Verification items for the finished model (mm, model axes). Face numbers are marked on the shaded views. A direction names the side the tool comes from. Coordinates: 2 decimals unless noted, no trailing zeros. Write each loop counter-clockwise with the first axis right and the second up, starting at its lowest first coordinate (ties: lowest second). Pieces come first, ordered by that corner, then holes. Notation, with made-up numbers: (50.25, -23.5) -> (106.25, -23.5) arc R25 ccw to (106.25, 4.5) -> close; hole circle Ø11 at (63, 11). An arc over 180 degrees is marked (long way). Answer in a Markdown table with one row per item.
```python
from build123d import *

# Parameters (mm, degrees)
SKETCH_1_R      = 5
SKETCH_1_R_2    = 3
EXTRUDE_1_DEPTH = 3
EXTRUDE_START   = -0.6
SKETCH_2_R      = 5.6
SKETCH_2_R_2    = 3
EXTRUDE_2_DEPTH = 0.6
FILLET_1_R      = 0.1


with BuildPart() as part:
    # ｽｹｯﾁ1 → ﾎﾞｽ - 押し出し1 (new body)
    with BuildSketch(Plane.XY):
        Circle(SKETCH_1_R)
        Circle(SKETCH_1_R_2, mode=Mode.SUBTRACT)
    extrude(amount=EXTRUDE_1_DEPTH)

    # ｽｹｯﾁ2 → ﾎﾞｽ - 押し出し2 (add)
    with BuildSketch(Plane.XY.offset(3).offset(EXTRUDE_START)):
        Circle(SKETCH_2_R)
        Circle(SKETCH_2_R_2, mode=Mode.SUBTRACT)
    extrude(amount=EXTRUDE_2_DEPTH)

    # ﾌｨﾚｯﾄ1
    fillet_1_edges = [part.edges().sort_by_distance(p)[0] for p in [
        (-5, 0, 0),
        (-3, 0, 0),
        (-3, 0, 3),
    ]]
    fillet(fillet_1_edges, radius=FILLET_1_R)


solid = part.part
```
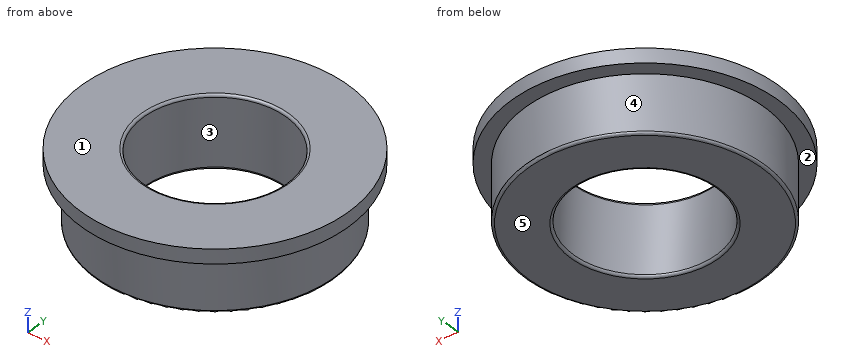
1. Sectioned sample at C-C, the plane z = 2.55. Record the cut outline in (x, y).
Findings below:
| item | result |
|---|---|
| outline | circle Ø11.2 at (0, 0); hole circle Ø6 at (0, 0) |
2. Access from +Z, -Z, +X, -X, +Y, -Y to the whole of each face (thin tool, end or side, straight path). Record for the marked faces 1 and 2.
Findings below:
| item | result |
|---|---|
| face 1 | +Z, +X, -X, +Y, -Y |
| face 2 | -Z |
3. Sectioned sample at A-A, the plane x = 0. Record the cut outline in (y, z), and give its area (3 significant figures).
Findings below:
| item | result |
|---|---|
| outline | (-5.6, 2.4) -> (-5, 2.4) -> (-5, 0.1) arc R0.1 ccw to (-4.9, 0) -> (-3.1, 0) arc R0.1 ccw to (-3, 0.1) -> (-3, 2.9) arc R0.1 ccw to (-3.1, 3) -> (-5.6, 3) -> close; (3, 0.1) arc R0.1 ccw to (3.1, 0) -> (4.9, 0) arc R0.1 ccw to (5, 0.1) -> (5, 2.4) -> (5.6, 2.4) -> (5.6, 3) -> (3.1, 3) arc R0.1 ccw to (3, 2.9) -> close |
| area | 12.7 mm² |
4. Release check for a two-part mould opening along X. For the marked faces 3, 4 and 5 record: released by +X, released by -X, zero draft, split by the parting line, or undercut.
Findings below:
| item | result |
|---|---|
| face 3 | undercut |
| face 4 | split by the parting line |
| face 5 | zero draft |
5. Sectioned sample at D-D, the plane z = 1.95. Record the cut outline in (x, y).
Findings below:
| item | result |
|---|---|
| outline | circle Ø10 at (0, 0); hole circle Ø6 at (0, 0) |
6. Go/stop test with flat-tipped pins: pin 1 (6 mm diameter, centred on x = 3.5, y = 0, fed in from -Z); pin 2 (4 mm diameter, centred on x = 0, y = -0.5, fed in from +Z) (3 decimals); pin 3 (1 mm diameter, centred on y = -1.5, z = 1, fed in from -X); pin 4 (1.5 mm diameter, centred on y = -2, z = 2, fed in from -X). Record where each tip stops, or that it passes through.
Findings below:
| item | result |
|---|---|
| pin 1 | stops at z = 0 |
| pin 2 | passes through |
| pin 3 | stops at x = -4.9 |
| pin 4 | stops at x = -5.43 |
7. Material ranges on probe 1 along Y at (x, z) = (0, 0.8); probe 2 along Y at (x, z) = (-2, 2.8); probe 3 along X at (y, z) = (-0.25, 1.35), recorded low to high. Write a range as from..to.
Findings below:
| item | result |
|---|---|
| probe 1 | y = -5..-3, 3..5 |
| probe 2 | y = -5.23..-2.24, 2.24..5.23 |
| probe 3 | x = -4.99..-2.99, 2.99..4.99 |
